Build history of the part. All positions in model axes, mm. Face numbers are marked on the shaded views. Give positions to 0.01 mm unless a question says otherwise; leave off trailing zeros. Order: outer loops, then holes, each group sorted by start corner. A loop starts at its lowest first (then second) coordinate and runs counter-clockwise, first axis right, second up. Notation, with made-up numbers: (19.5, 71.25) - (41.5, 71.25) arc R18 cw to (41.5, 83.25) - close; hole circle Ø4 at (-21.5, 57). An arc over 180 degrees is marked (long way). Use a Markdown table: item, result.
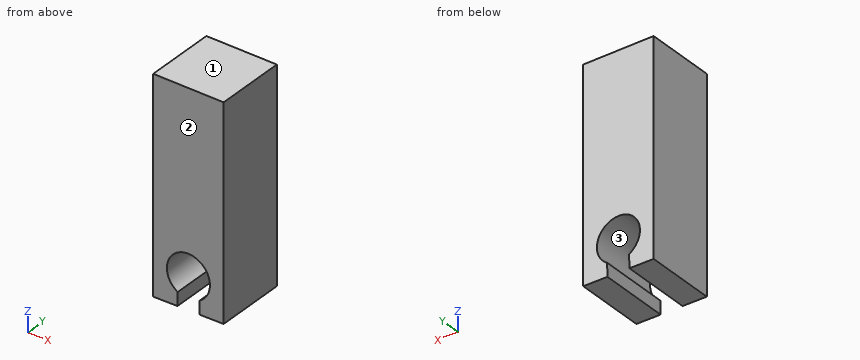
from build123d import *

# Parameters (mm, degrees)
F1_DEPTH = 50


with BuildPart() as f1:
    # F0 (on Front) → F1 (new body)
    with BuildSketch(Plane.XZ):
        with BuildLine():
            Line((33.008534, 10.347258), (32.810526, 0.825341))
            Line((32.810526, 0.825341), (49.995198, 1.100471))
            Line((49.995198, 1.100471), (49.995198, 150))
            Line((49.995198, 150), (0, 150))
            Line((0, 150), (0, 0.300038))
            Line((0, 0.300038), (17.201957, 0.575445))
            Line((17.201957, 0.575445), (17.400121, 10.104875))
            ThreePointArc((17.400121, 10.104875), (24.762435, 38.682031), (33.008534, 10.347258))
        make_face()
    extrude(amount=F1_DEPTH)


solid = f1.part
1) Pin check, flat tips, straight feed: P1, Ø4, axis at x = 7, y = -24, coming from the -Z side; P2, Ø10, axis at x = 20.5, y = -33, coming from the -Z side; P3, Ø10, axis at x = 37, y = -9.5, coming from the -Z side. Stop position of each tip, or through.
Computed:
| item | result |
|---|---|
| P1 | stops at z = 0.38 |
| P2 | stops at z = 0.55 |
| P3 | stops at z = 0.83 |
2) Slice it at A-A (x = 36). Write the cut outline in (y, z), and give its area (3 significant figures).
Computed:
| item | result |
|---|---|
| outline | (-50, 0.88) - (0, 0.88) - (0, 12.75) - (-50, 12.75) - close; (-50, 34.02) - (0, 34.02) - (0, 150) - (-50, 150) - close |
| area | 6,390 mm² |
3) Slice it at D-D (x = 25). Write the cut outline in (y, z).
Computed:
| item | result |
|---|---|
| outline | (-50, 38.68) - (0, 38.68) - (0, 150) - (-50, 150) - close |
4) Slice it at B-B (y = -27). Write the cut outline in (x, z).
Computed:
| item | result |
|---|---|
| outline | (0, 0.3) - (17.2, 0.58) - (17.4, 10.1) arc R15.3 cw (long way) to (33.01, 10.35) - (32.81, 0.83) - (50, 1.1) - (50, 150) - (0, 150) - close |
5) Slice it at C-C (z = 17.5). Write the cut outline in (x, y).
Computed:
| item | result |
|---|---|
| outline | (0, -50) - (10.88, -50) - (10.88, 0) - (0, 0) - close; (39.12, -50) - (50, -50) - (50, 0) - (39.12, 0) - close |
6) Wall check: line 1 (Z direction, x = 25, y = -38); line 2 (X direction, y = -18.5, z = 34); line 3 (Z direction, x = 11, y = -30). Give the ranges that are in metal, low to high. Write a range as from..to.
Computed:
| item | result |
|---|---|
| line 1 | z = 38.68..150 |
| line 2 | x = 0..13.98, 36.02..50 |
| line 3 | z = 0.48..17.21, 29.56..150 |
7) Two-plate mould, pull along Z, no slides. Class the marked faces 1, 2 and 3: +Z half, -Z half, draft (parallel to the pull), parting line (faces both ways), or undercut.
Computed:
| item | result |
|---|---|
| face 1 | +Z half |
| face 2 | draft |
| face 3 | undercut |
